Source: CAD feature listing. Evaluate the final solid. Frame: model axes, mm. Face numbers are marked on the shaded views. Give positions to 0.01 mm unless a question says otherwise; leave off trailing zeros. Loops run counter-clockwise (first coordinate to the right, second up) from the corner with the lowest first, then second, coordinate; pieces in that order, holes last.
```python
from build123d import *

# Parameters (mm, degrees)
SK_CRANK_PLATE_R   = 1.7
SK_CRANK_PLATE_R_2 = 2.5
CRANK_PLATE_DEPTH  = 6
SK_PILOT_RECESS_R  = 17.15
PILOT_RECESS_DEPTH = 2.2


with BuildPart() as part:
    # SK_Crank_Plate → Crank_Plate (new body)
    with BuildSketch(Plane.XY):
        Polygon((-59, -9), (-19.6, -28), (19.6, -28), (28, 0), (19.6, 28), (-19.6, 28), (-59, 9), align=None)
        with Locations((23, 0)):
            Circle(SK_CRANK_PLATE_R, mode=Mode.SUBTRACT)
        with Locations((11.5, 19.918584287)):
            Circle(SK_CRANK_PLATE_R, mode=Mode.SUBTRACT)
        with Locations((-11.5, 19.918584287)):
            Circle(SK_CRANK_PLATE_R, mode=Mode.SUBTRACT)
        with Locations((-23, 0)):
            Circle(SK_CRANK_PLATE_R, mode=Mode.SUBTRACT)
        with Locations((-11.5, -19.918584287)):
            Circle(SK_CRANK_PLATE_R, mode=Mode.SUBTRACT)
        with Locations((11.5, -19.918584287)):
            Circle(SK_CRANK_PLATE_R, mode=Mode.SUBTRACT)
        with Locations((-50, 0)):
            Circle(SK_CRANK_PLATE_R_2, mode=Mode.SUBTRACT)
    extrude(amount=CRANK_PLATE_DEPTH)

    # SK_Pilot_Recess → Pilot_Recess (cut)
    with BuildSketch(Plane.XY):
        Circle(SK_PILOT_RECESS_R)
    extrude(amount=PILOT_RECESS_DEPTH, mode=Mode.SUBTRACT)


solid = part.part
```
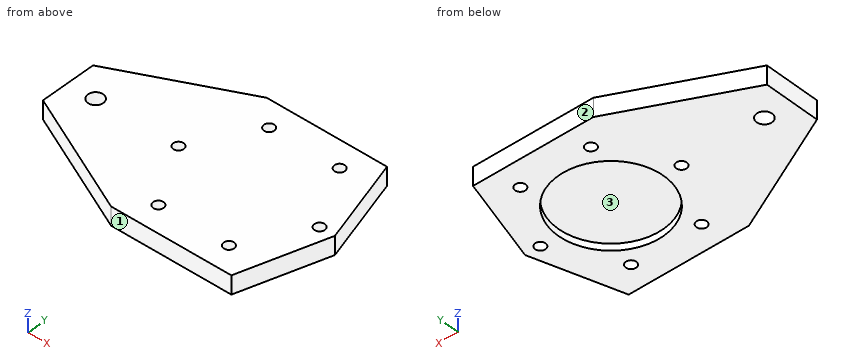
(1) Section B-B, the plane x = 0. Return the cut outline in (y, z).
A:
outline: (-28, 0) - (-17.15, 0) - (-17.15, 2.2) - (17.15, 2.2) - (17.15, 0) - (28, 0) - (28, 6) - (-28, 6) - close
(2) First-contact query: pin 1 (2 mm diameter, centred on x = -43, z = 1, fed in from +Y); pin 2 (17 mm diameter, centred on x = 3, y = -1, fed in from -Z); pin 3 (3 mm diameter, centred on x = 11.5, y = -19.92, fed in from +Z); pin 4 (3 mm diameter, centred on y = 6, z = 1.5, fed in from +X). Flat tips, straight axial feed; report the tip coordinate or a pass-through.
A:
pin 1: stops at y = 17.2
pin 2: stops at z = 2.2
pin 3: passes through
pin 4: stops at x = 26.65
(3) Section D-D, the plane z = 1. Count the separate pieces of the cut face and the enclosed holes in it, then the cut area to 3 significant figures.
A:
separate pieces: 1
enclosed holes: 8
area: 2,890 mm2
(4) Ray query, line 1 along Y through (x, z) = (-11.5, 3.3); line 2 along X through (y, z) = (-1.5, 2.7); line 3 along X through (y, z) = (1, 5.05). Return the intervals inside material, ascending.
A:
line 1: y = -28 to -21.62, -18.22 to 18.22, 21.62 to 28
line 2: x = -59 to -52, -48 to -23.8, -22.2 to 22.2, 23.8 to 27.55
line 3: x = -59 to -52.29, -47.71 to -24.37, -21.63 to 21.63, 24.37 to 27.7
(5) Section C-C, the plane z = 4.9. Return the cut outline in (x, y).
A:
outline: (-59, -9) - (-19.6, -28) - (19.6, -28) - (28, 0) - (19.6, 28) - (-19.6, 28) - (-59, 9) - close; hole circle Ø5 at (-50, 0); hole circle Ø3.4 at (-23, 0); hole circle Ø3.4 at (-11.5, -19.92); hole circle Ø3.4 at (-11.5, 19.92); hole circle Ø3.4 at (11.5, -19.92); hole circle Ø3.4 at (11.5, 19.92); hole circle Ø3.4 at (23, 0)
(6) Mould query, pull axis Y, two halves, no side actions, for the marked faces 1, 2 and 3. Classes: pulls with the +Y half, pulls with the -Y half, needs draft (parallel to the pull), parting line crosses it, or undercut.
A:
face 1: pulls with the -Y half
face 2: pulls with the +Y half
face 3: undercut
(7) Section A-A, the plane x = -48.5. Return the cut outline in (y, z), then the cut area to 3 significant figures.
A:
outline: (-14.06, 0) - (-2, 0) - (-2, 6) - (-14.06, 6) - close; (2, 0) - (14.06, 0) - (14.06, 6) - (2, 6) - close
area: 145 mm2
